Verification items for this drawing (mm, ordinates from the low corner). A direction names the side the tool comes from. Round coordinates to 2 decimals unless told otherwise and drop trailing zeros. Loops run counter-clockwise (first coordinate to the right, second up) from the corner with the lowest first, then second, coordinate; pieces in that order, holes last. Notation, with made-up numbers: (-4, 86.25) -> (6, 86.25) arc R20 ccw to (6, 90.25) -> close; hole circle Ø10 at (-5.5, -38). An arc over 180 degrees is marked (long way). Use a Markdown table: item, result. Add a question column.
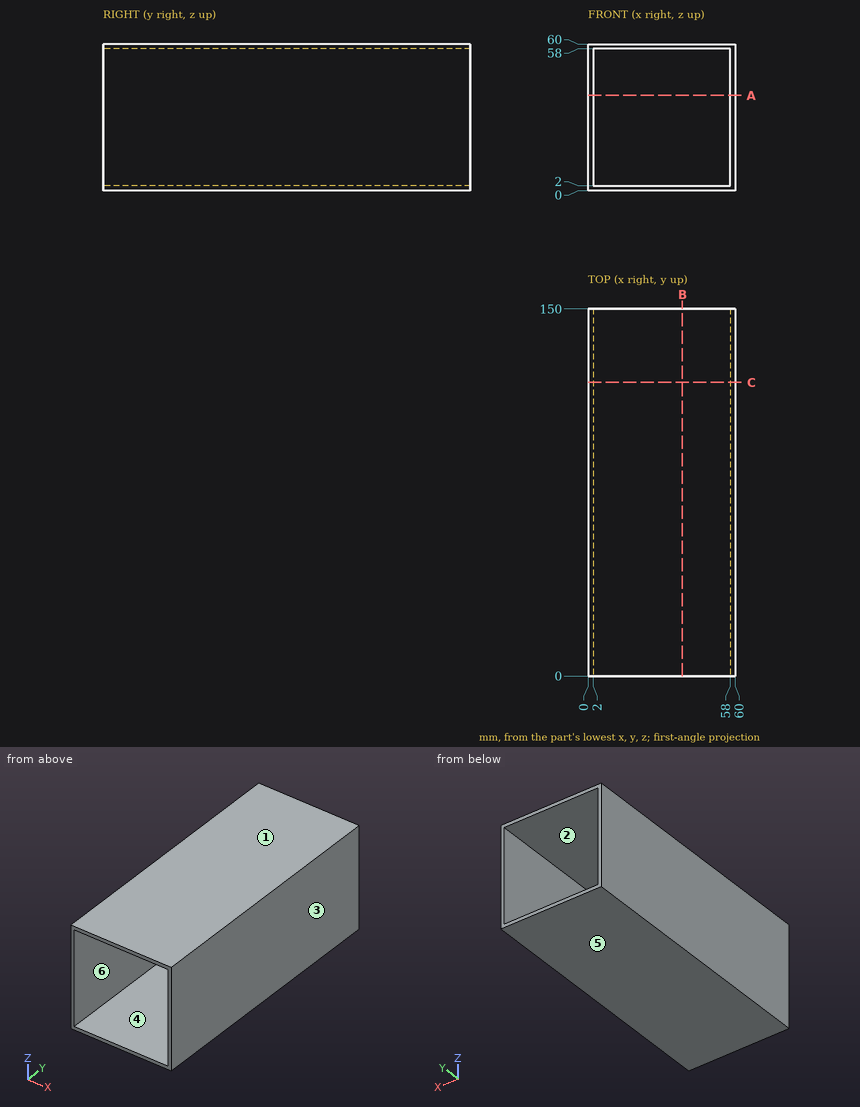
1) Release check for a two-part mould opening along X. For the marked faces 1, 2, 3 and 4 record: released by +X, released by -X, zero draft, split by the parting line, or undercut.
2) Sectioned sample at A-A on z = 39. Enter the section's corners in (x, y).
3) Thickness scan on line 1 (X direction, y = 131, z = 47). Record the ranges inside material, lowest first.
4) Sectioned sample at B-B on x = 38.5. Enter the section's corners in (y, z), then the cut area to 3 significant figures.
5) Sectioned sample at C-C on y = 120. Enter the section's corners in (x, z), then the cut area to 3 significant figures.
6) Access from +Z, -Z, +X, -X, +Y, -Y to the whole of each face (thin tool, end or side, straight path). Record for the marked faces 5 and 6.
Geometry results:
| question | item | result |
|---|---|---|
| 1 | face 1 | zero draft |
| 1 | face 2 | undercut |
| 1 | face 3 | released by +X |
| 1 | face 4 | undercut |
| 2 | outline | (0, 0) -> (2, 0) -> (2, 150) -> (0, 150) -> close; (58, 0) -> (60, 0) -> (60, 150) -> (58, 150) -> close |
| 3 | line 1 | 0 to 2, 58 to 60 |
| 4 | outline | (0, 0) -> (150, 0) -> (150, 2) -> (0, 2) -> close; (0, 58) -> (150, 58) -> (150, 60) -> (0, 60) -> close |
| 4 | area | 600 mm^2 |
| 5 | outline | (0, 0) -> (60, 0) -> (60, 60) -> (0, 60) -> close; hole (2, 2) -> (58, 2) -> (58, 58) -> (2, 58) -> close |
| 5 | area | 464 mm^2 |
| 6 | face 5 | -Z, +X, -X, +Y, -Y |
| 6 | face 6 | +Y, -Y |
